Geometry: see drawing. Coordinates: mm, zero at the bounding-box minimum. A direction names the side the tool comes from. Coordinates: 2 decimals unless noted, no trailing zeros. Loops run counter-clockwise (first coordinate to the right, second up) from the corner with the lowest first, then second, coordinate; pieces in that order, holes last.
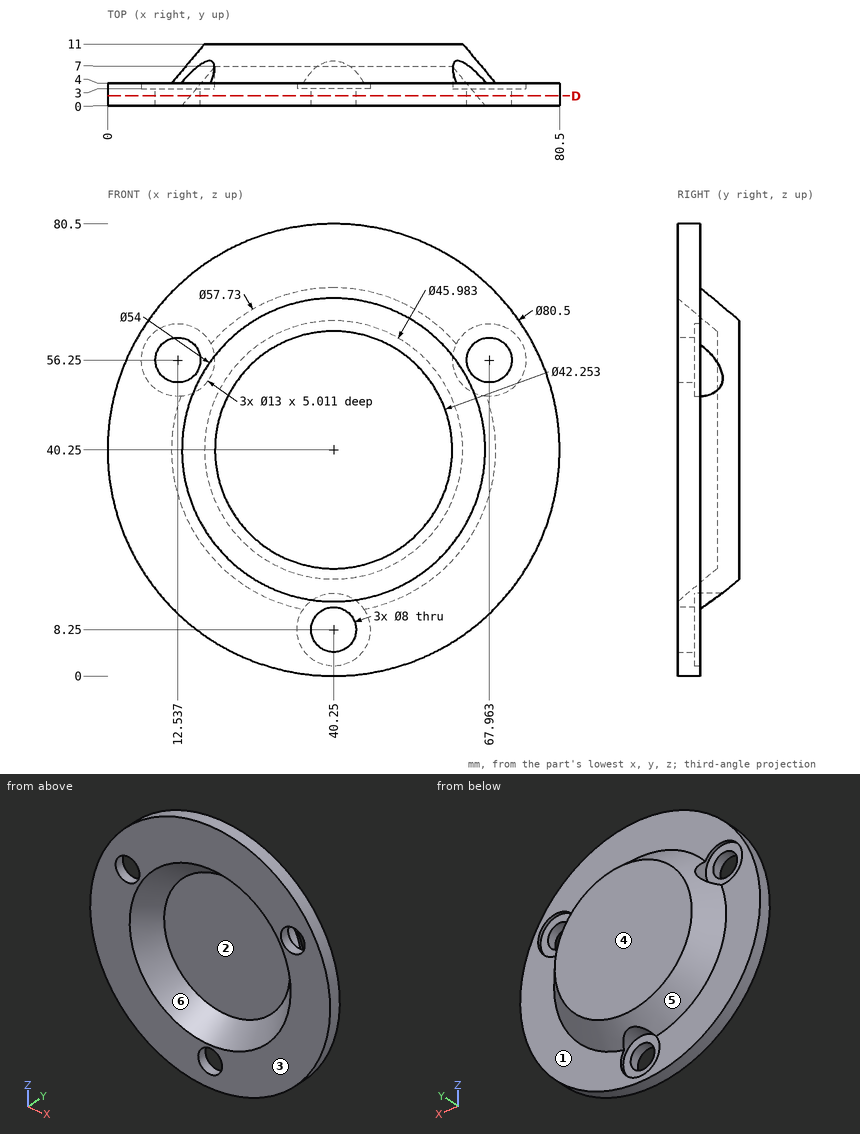
Item 1: Contact query for flat-ended pins moving along their axis: P1, Ø6, axis at x = 15, y = 5, coming from the +Z side; P2, Ø15, axis at x = 40.25, z = 8.25, coming from the +Y side; P3, Ø10.5, axis at x = 67.96, z = 56.25, coming from the +Y side. Output: stop coordinate, or through.
Result:
P1: stops at z = 73.68
P2: stops at y = 9.2
P3: stops at y = 3
Item 2: Line query: L1, parallel to X at y = 2.5, z = 58 (1 decimal); L2, parallel to Y at x = 7, z = 32; L3, parallel to Z at x = 11, y = 2.5 (1 decimal). Output: solid intervals per line, ascending.
Result:
L1: x = 4.1 to 8.9, 16.1 to 22.8, 57.7 to 64.4, 71.6 to 76.4
L2: y = 0 to 4
L3: z = 12.6 to 52.6, 59.9 to 67.9
Item 3: Mould query, pull axis Z, two halves, no side actions, for the marked faces 4, 5 and 6. Classes: +Z half, -Z half, draft (parallel to the pull), parting line (faces both ways), or undercut.
Result:
face 4: draft
face 5: parting line
face 6: undercut
Item 4: Reachability of the marked faces 1, 2 and 3 from +Z, -Z, +X, -X, +Y, -Y: full face, straight path, thin tool, end or side. Return the list, or none.
Result:
face 1: +Y
face 2: -Y
face 3: +Z, -Z, +X, -X, -Y
Item 5: Section query D-D (y = 1.75). Output: boundary loops of the cut face in (x, z), then the cut area to 3 significant figures.
Result:
outline: circle Ø80.5 at (40.25, 40.25); hole circle Ø8 at (12.54, 56.25); hole circle Ø51.06 at (40.25, 40.25); hole circle Ø8 at (40.25, 8.25); hole circle Ø8 at (67.96, 56.25)
area: 2,890 mm2
